Autodesk Inventor part; units mm, degrees
ref_plane "YZ Plane" through (0, 0, 0) normal (1, 0, 0) x (0, 1, 0)
ref_plane "XZ Plane" through (0, 0, 0) normal (0, 1, 0) x (-1, 0, 0)
ref_plane "XY Plane" through (0, 0, 0) normal (0, 0, 1) x (1, 0, 0)
sketch "Sketch1" plane through (0, 0, 0) normal (0, 1, 0) x (-1, 0, 0)
  line L0 (50.5, 51.5) -> (-50.5, 51.5)
  line L1 (-50.5, 51.5) -> (-50.5, -51.5)
  line L2 (-50.5, -51.5) -> (50.5, -51.5)
  line L3 (50.5, -51.5) -> (50.5, 51.5)
  line L4 (50.5, 51.5) -> (-50.5, -51.5) construction
  line L5 (-50.5, 51.5) -> (50.5, -51.5) construction
  line L6 (48.4022, -49.4) -> (-47.3, -49.4)
  line L7 (-47.3, 49.4022) -> (48.4022, 49.4022)
  line L8 (48.4022, 49.4022) -> (48.4022, -49.4)
  line L9 (-47.3, -47.9892) -> (-47.3, 42.6215)
  line L10 (-47.3, -47.9892) -> (-47.3, -49.4)
  line L11 (-47.3, 42.6215) -> (-47.3, 49.4022)
  line L12 (46.9022, -47.9) -> (-45.8, -47.9)
  line L13 (-45.8, -47.9) -> (-45.8, 42.6215)
  line L14 (-45.8, 42.6215) -> (-45.8, 47.9022)
  line L15 (-45.8, 47.9022) -> (46.9022, 47.9022)
  line L16 (46.9022, 47.9022) -> (46.9022, -47.9)
  point P0 (0, 0)
  dimension "d0" = 101
  dimension "d1" = 103
  dimension "d2" = 2.1
  dimension "d3" = 3.2
  dimension "d4" = 1.5
extrude "Extrusion1" add sketch "Sketch1" along normal blind 1.5 contours L3 L2 L1 L0 | L6 L10 L9 L11 L7 L8 | L12 L13 L14 L15 L16
extrude "Extrusion2" add sketch "Sketch1" along normal blind 4 contours L6 L10 L9 L11 L7 L8
sketch "Sketch2" plane through (0, 1.5, 0) normal (0, 1, 0) x (1, 0, 0)
  circle A0 centre (0, 0) radius 2.1
  dimension "d9" = 4.2
extrude "Extrusion3" cut sketch "Sketch2" against normal blind 4
properties part number "TAPA GENERAL_3DPrint"
Can you work these out from the model? Positions are in its coordinate system, mm. A direction names the side the tool comes from. Coordinates: 2 decimals unless noted, no trailing zeros. Order: outer loops, then holes, each group sorted by start corner. A loop starts at its lowest first (then second) coordinate and runs counter-clockwise, first axis right, second up. Notation, with made-up numbers: (-18.5, -38) -> (-0.5, -38) arc R23 cw to (-0.5, -6) -> close; hole circle Ø10 at (66, 24). An arc over 180 degrees is marked (long way). Write each question's results on one line, items separated by ' | '.
Item 1: Which directions (+Z, -Z, +X, -X, +Y, -Y) give clear straight access to the entire face, cutting with the end or side of a thin tool? Please do faces 4 (the face through (2.003, 0.76, -0.631)), 5 (the face through (0, 3, 49.402)), 6 (the face through (-48.402, 3, 1)), 7 (the face through (-1, 3, -47.9)), 8 (the face through (47.3, 3, -1)).
Results are:
face 4: +Y, -Y | face 5: +Z, +X, -X, +Y | face 6: +Z, -Z, -X, +Y | face 7: +Y | face 8: +Z, -Z, +X, +Y
Item 2: I want a section at A-A, the plane y = 2.2. Write out the boundary of the cut face in (x, z).
Results are:
outline: (-48.4, -49.4) -> (47.3, -49.4) -> (47.3, 49.4) -> (-48.4, 49.4) -> close; hole (-46.9, -47.9) -> (45.8, -47.9) -> (45.8, 47.9) -> (-46.9, 47.9) -> close
Item 3: I want a section at D-D, the plane x = -22.5. Write out the boundary of the cut face in (y, z).
Results are:
outline: (0, -51.5) -> (1.5, -51.5) -> (1.5, -49.4) -> (4, -49.4) -> (4, -47.9) -> (1.5, -47.9) -> (1.5, 47.9) -> (4, 47.9) -> (4, 49.4) -> (1.5, 49.4) -> (1.5, 51.5) -> (0, 51.5) -> close
Item 4: If I drill on line 1 along Z through (x, y) = (-28, 2.4); line 2 along Z through (x, y) = (0, 0.9); line 3 along X through (y, z) = (0.9, 0), over which ranges is the centre line in solid material (lowest first)?
Results are:
line 1: -49.4 to -47.9, 47.9 to 49.4 | line 2: -51.5 to -2.1, 2.1 to 51.5 | line 3: -50.5 to -2.1, 2.1 to 50.5
Item 5: I want a section at C-C, the plane z = 0. Write out the boundary of the cut face in (x, y).
Results are:
outline: (-50.5, 0) -> (-2.1, 0) -> (-2.1, 1.5) -> (-46.9, 1.5) -> (-46.9, 4) -> (-48.4, 4) -> (-48.4, 1.5) -> (-50.5, 1.5) -> close; (2.1, 0) -> (50.5, 0) -> (50.5, 1.5) -> (47.3, 1.5) -> (47.3, 4) -> (45.8, 4) -> (45.8, 1.5) -> (2.1, 1.5) -> close
Item 6: I'm going to push flat-ended pins straight in: pin 1 Ø1.2 at (y, z) = (3, 1) entering from -X; pin 2 Ø0.8 at (y, z) = (3, 11) entering from +X; pin 3 Ø2.5 at (x, z) = (0, 0) entering from -Y; pin 4 Ø1.2 at (x, y) = (5, 2.5) entering from -Z. Where does each tip first touch, or does it pass through?
Results are:
pin 1: x = -48.4 | pin 2: x = 47.3 | pin 3: through | pin 4: z = -49.4
Item 7: I want a section at B-B, the plane x = 0. Write out the boundary of the cut face in (y, z).
Results are:
outline: (0, -51.5) -> (1.5, -51.5) -> (1.5, -49.4) -> (4, -49.4) -> (4, -47.9) -> (1.5, -47.9) -> (1.5, -2.1) -> (0, -2.1) -> close; (0, 2.1) -> (1.5, 2.1) -> (1.5, 47.9) -> (4, 47.9) -> (4, 49.4) -> (1.5, 49.4) -> (1.5, 51.5) -> (0, 51.5) -> close
Item 8: If we mould it in two halves opening along Z, with no side actions, what happens to faces 1 (the face through (-11, 0, 1)), 2 (the face through (-1, 3, -49.4)), 3 (the face through (-46.902, 3, 1))? For each: +Z half, -Z half, draft (parallel to the pull), parting line (faces both ways), or undercut.
Results are:
face 1: draft | face 2: -Z half | face 3: undercut
